```python
from build123d import *

# Parameters (mm, degrees)
F0_W         = 50
F0_H         = 35
F1_DEPTH     = 7.6
F2_W         = 50
F2_H         = 25
F3_DEPTH     = 5
F4_T4_DEPTH  = 50
F4_T9_DEPTH  = 50
F4_T11_DEPTH = 83.9462154412
F5_W         = 40
F5_H         = 5
F6_DEPTH     = 2.6
F7_R         = 2.49999


# Not quite as in the source:
# - a fillet or chamfer that OpenCascade refuses, or shapes differently, is made with other operations: its cross-section is extruded or revolved along the edge and cut away or added
# - a fillet or chamfer is up to 0.001 mm smaller than in the source, because OpenCascade refuses the exact size


with BuildPart() as f1:
    # F0 (on Top) → F1 (new body)
    with BuildSketch(Plane.XY):
        Rectangle(F0_W, F0_H)
    extrude(amount=F1_DEPTH)

    # F2 (on face) → F3 (cut)
    with BuildSketch(Plane.XY.offset(7.6)):
        Rectangle(F2_W, F2_H)
    extrude(amount=-F3_DEPTH, mode=Mode.SUBTRACT)

    # F4: chamfer of 6.6 on 4 edges, made by hand


with BuildPart() as f4_tool2:
    # F4_s3 → F4_t4 (new body)
    with BuildSketch(Plane.YZ.offset(25)):
        Polygon((5.9, 2.6), (12.5, 9.2), (12.5, 2.6), align=None)
    extrude(amount=-F4_T4_DEPTH)

    split(bisect_by=Plane.XY.offset(7.6), keep=Keep.BOTTOM)


with BuildPart() as f1_1:
    add(f1.part)

    # F4_t1: union F4_tool2
    add(f4_tool2.part)


with BuildPart() as f4_tool7:
    # F4_s8 → F4_t9 (new body)
    with BuildSketch(Plane.YZ.offset(-25)):
        Polygon((-12.5, 9.2), (-5.9, 2.6), (-12.5, 2.6), align=None)
    extrude(amount=F4_T9_DEPTH)

    split(bisect_by=Plane.XY.offset(7.6), keep=Keep.BOTTOM)


with BuildPart() as f1_2:
    add(f1_1.part)

    # F4_t6: union F4_tool7
    add(f4_tool7.part)

    # F4_s12 → F4_t11 (cut)
    with BuildSketch(Plane.YZ.offset(-41.9731077206)):
        Polygon((17.5, 6.6), (10.9, 0), (17.5, 0), align=None)
        Polygon((-17.5, 6.6), (-10.9, 0), (-17.5, 0), align=None)
    extrude(amount=F4_T11_DEPTH, mode=Mode.SUBTRACT)

    # F5 (on face) → F6 (cut, through all)
    with BuildSketch(Plane.XY.offset(2.6)):
        Rectangle(F5_W, F5_H)
    extrude(amount=-F6_DEPTH, mode=Mode.SUBTRACT)

    # F7 (radius 2.5 in the source; OpenCascade refuses exactly that, so slightly less here)
    f7_edges = [f1_2.edges().sort_by_distance(p)[0] for p in [
        (-20, -2.5, 1.3),
        (-20, 2.5, 1.3),
        (20, 2.5, 1.3),
        (20, -2.5, 1.3),
    ]]
    fillet(f7_edges, radius=F7_R)


solid = f1_2.part
```
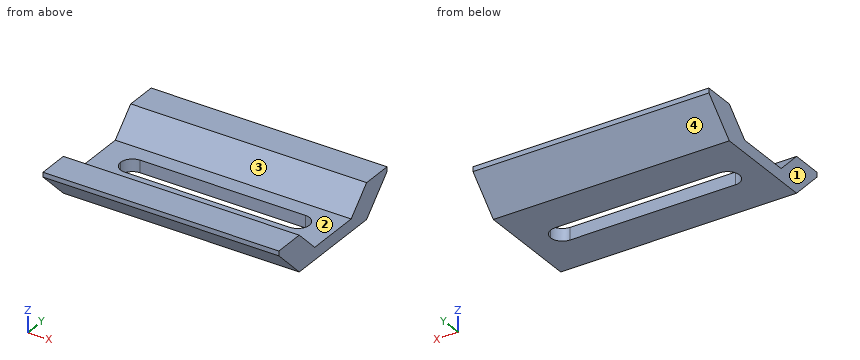
The model under review builds one solid part; all positions refer to its coordinate system, in mm. Face numbers are marked on the shaded views. Give positions to 0.01 mm unless a question says otherwise; leave off trailing zeros. Order: outer loops, then holes, each group sorted by start corner. A loop starts at its lowest first (then second) coordinate and runs counter-clockwise, first axis right, second up. Notation, with made-up numbers: (73.5, 43) - (123.5, 43) arc R13 ccw to (123.5, 58) - close; hole circle Ø9 at (74, 47.25). An arc over 180 degrees is marked (long way). Use CSV: the item, a comma, the result in double quotes. Start each with the question number.
Q1. We need section D-D, the plane y = 14.5. Write out the cut boundary in (x, z).
Q2. The part is to be moulded in two halves that separate along Y. For the marked faces 1, 2, 3 and 4, say which applies: +Y half, -Y half, draft (parallel to the pull), parting line (faces both ways), or undercut.
Q3. We need section C-C, the plane z = 5. Write out the cut boundary in (x, y).
Q4. To check wall thickness, follow line 1 along Y through (x, z) = (11.5, 6.25); line 2 along Y through (x, z) = (-13, 3.5); line 3 along Z through (x, y) = (16, 5). State the ranges of each line that lie inside material, in increasing order. Write a range as [from, to].
Q5. Clearance check with flat-ended pins moving along their axes: pin 1 Ø5 at (x, y) = (-2.5, -6.5) entering from +Z; pin 2 Ø0.8 at (x, z) = (-2, 1) entering from +Y; pin 3 Ø13 at (x, y) = (-2, -1.5) entering from +Z. State where each tip first meets the part, or that it passes through.
Q6. We need section A-A, the plane x = -8.5. Write out the cut boundary in (y, z), and give its area (3 significant figures).
Outcome:
1,outline,"(-25, 3.6) - (25, 3.6) - (25, 7.6) - (-25, 7.6) - close"
2,face 1,"draft"
2,face 2,"undercut"
2,face 3,"undercut"
2,face 4,"+Y half"
3,outline,"(-25, -15.9) - (25, -15.9) - (25, -8.3) - (-25, -8.3) - close; (-25, 8.3) - (25, 8.3) - (25, 15.9) - (-25, 15.9) - close"
4,line 1,"y = [-17.15, -9.55], [9.55, 17.15]"
4,line 2,"y = [-14.4, -6.8], [6.8, 14.4]"
4,line 3,"z = [0, 2.6]"
5,pin 1,"stops at z = 5.7"
5,pin 2,"stops at y = 12.3"
5,pin 3,"stops at z = 4.7"
6,outline,"(-17.5, 6.6) - (-10.9, 0) - (-2.5, 0) - (-2.5, 2.6) - (-5.9, 2.6) - (-10.9, 7.6) - (-17.5, 7.6) - close; (2.5, 0) - (10.9, 0) - (17.5, 6.6) - (17.5, 7.6) - (10.9, 7.6) - (5.9, 2.6) - (2.5, 2.6) - close"
6,area,"125 mm^2"
